Work out the finished part from the listing and answer in its coordinate system (mm). Face numbers are marked on the shaded views. A direction names the side the tool comes from. Round coordinates to 2 decimals unless told otherwise and drop trailing zeros. Write each loop counter-clockwise with the first axis right and the second up, starting at its lowest first coordinate (ties: lowest second). Pieces come first, ordered by that corner, then holes. Notation, with made-up numbers: (67, -23.5) -> (80, -23.5) arc R31 cw to (80, 6.5) -> close; hole circle Ø8 at (14.5, 40). An arc over 180 degrees is marked (long way). One line per item, written item: value.
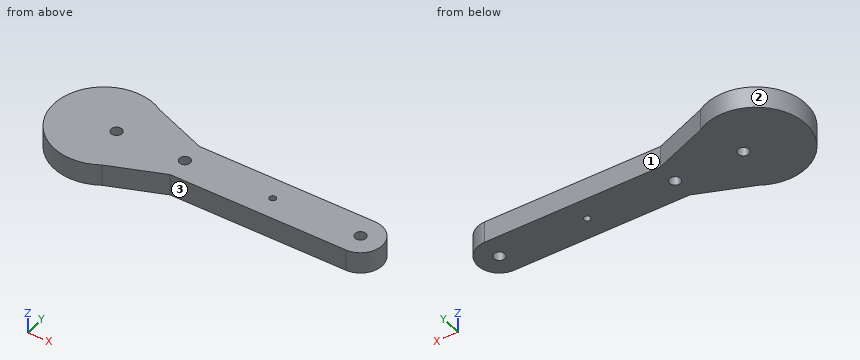
```python
from build123d import *

# Parameters (mm, degrees)
ESQUISSE1_R        = 2.5
ESQUISSE1_R_2      = 1.5
BOSS_EXTRU_1_DEPTH = 10


with BuildPart() as part:
    # Esquisse1 → Boss.-Extru.1 (new body)
    with BuildSketch(Plane.XY):
        with BuildLine():
            Line((0, 0), (80, 0))
            ThreePointArc((80, 0), (90, 10), (80, 20))
            Line((80, 20), (0, 20))
            Line((0, 20), (-24.667286758, 29.658401944))
            ThreePointArc((-24.667286758, 29.658401944), (-59.912850456, 10), (-24.667286758, -9.658401944))
            Line((-24.667286758, -9.658401944), (0, 0))
        make_face()
        with Locations((0, 10)):
            Circle(ESQUISSE1_R, mode=Mode.SUBTRACT)
        with Locations((80, 10)):
            Circle(ESQUISSE1_R, mode=Mode.SUBTRACT)
        with Locations((-31.091119471, 10)):
            Circle(ESQUISSE1_R, mode=Mode.SUBTRACT)
        with Locations((40, 10)):
            Circle(ESQUISSE1_R_2, mode=Mode.SUBTRACT)
    extrude(amount=BOSS_EXTRU_1_DEPTH)


solid = part.part
```
(1) Find section C-C on z = 7.25. Give the vertices of the cut face in (x, y), plus the area to 3 significant figures.
Reported:
outline: (-24.67, -9.66) -> (0, 0) -> (80, 0) arc R10 ccw to (80, 20) -> (0, 20) -> (-24.67, 29.66) arc R23.11 ccw (long way) to start; hole circle Ø5 at (-31.09, 10); hole circle Ø5 at (0, 10); hole circle Ø3 at (40, 10); hole circle Ø5 at (80, 10)
area: 3,800 mm2
(2) A tool of negligible diameter and unlimited length cuts with its end or side. For the marked faces 1, 2 and 3, from which of +Z, -Z, +X, -X, +Y, -Y can it reach the whole face along a straight path? Write none if from no direction.
Reported:
face 1: +Z, -Z, +X, +Y
face 2: +Z, -Z
face 3: +Z, -Z, +X, -Y
(3) Find section B-B on y = 10. Give the vertices of the cut face in (x, z), plus the area to 3 significant figures.
Reported:
outline: (-59.91, 0) -> (-33.59, 0) -> (-33.59, 10) -> (-59.91, 10) -> close; (-28.59, 0) -> (-2.5, 0) -> (-2.5, 10) -> (-28.59, 10) -> close; (2.5, 0) -> (38.5, 0) -> (38.5, 10) -> (2.5, 10) -> close; (41.5, 0) -> (77.5, 0) -> (77.5, 10) -> (41.5, 10) -> close; (82.5, 0) -> (90, 0) -> (90, 10) -> (82.5, 10) -> close
area: 1,320 mm2
(4) Find section D-D on x = 19. Give the vertices of the cut face in (y, z).
Reported:
outline: (0, 0) -> (20, 0) -> (20, 10) -> (0, 10) -> close
(5) Flat-ended cylindrical pins translate along their axes: pin 1 Ø6 at (x, z) = (-23.5, 5) entering from +Y; pin 2 Ø1 at (x, z) = (-7.5, 6.5) entering from +Y; pin 3 Ø5 at (x, z) = (54, 3.5) entering from +Y. Find the tip coordinate at first contact, or state that the pin passes through.
Reported:
pin 1: stops at y = 30.68
pin 2: stops at y = 23.13
pin 3: stops at y = 20
(6) Consider probe 1 along Y at (x, z) = (80, 7.75); probe 2 along X at (y, z) = (9.5, 3); probe 3 along Y at (x, z) = (27.5, 8.25). Determine where each line is inside the solid, lowest interval first.
Reported:
probe 1: y = 0 to 7.5, 12.5 to 20
probe 2: x = -59.91 to -33.54, -28.64 to -2.45, 2.45 to 38.59, 41.41 to 77.55, 82.45 to 89.99
probe 3: y = 0 to 20
(7) Find section A-A on x = 40. Give the vertices of the cut face in (y, z).
Reported:
outline: (0, 0) -> (8.5, 0) -> (8.5, 10) -> (0, 10) -> close; (11.5, 0) -> (20, 0) -> (20, 10) -> (11.5, 10) -> close
